```python
from build123d import *

# Parameters (mm, degrees)
SKETCH1_R           = 30
BOSS_EXTRUDE1_DEPTH = 3
SKETCH2_R           = 10
BOSS_EXTRUDE2_DEPTH = 2
SKETCH3_W           = 10
SKETCH3_H           = 15
BOSS_EXTRUDE3_DEPTH = 10
CUT_EXTRUDE1_START  = -1.5
SKETCH4_W           = 10
SKETCH4_H           = 10
CUT_EXTRUDE1_DEPTH  = 12
SKETCH5_R           = 2.5
CUT_EXTRUDE2_DEPTH  = 50.751884386


with BuildPart() as part:
    # Sketch1 → Boss-Extrude1 (new body)
    with BuildSketch(Plane(origin=(0, 0, 0), x_dir=(1, 0, 0), z_dir=(0, 1, 0))):
        with Locations(Location((0, 0, 0), (0, 0, 270))):
            Circle(SKETCH1_R)
    extrude(amount=BOSS_EXTRUDE1_DEPTH)

    # Sketch2 → Boss-Extrude2 (add)
    with BuildSketch(Plane(origin=(0, 3, 0), x_dir=(1, 0, 0), z_dir=(0, 1, 0))):
        with Locations(Location((0, 0, 0), (0, 0, 270))):
            Circle(SKETCH2_R)
    extrude(amount=BOSS_EXTRUDE2_DEPTH)

    # Sketch3 → Boss-Extrude3 (add)
    with BuildSketch(Plane(origin=(0, 3, 0), x_dir=(1, 0, 0), z_dir=(0, 1, 0))):
        with Locations((-20, 0)):
            Rectangle(SKETCH3_W, SKETCH3_H)
        with Locations((20, 0)):
            Rectangle(SKETCH3_W, SKETCH3_H)
    extrude(amount=BOSS_EXTRUDE3_DEPTH)

    # Sketch4 → Cut-Extrude1 (cut)
    with BuildSketch(Plane.XY.offset(7.5).offset(CUT_EXTRUDE1_START)):
        with Locations((-20, 8)):
            Rectangle(SKETCH4_W, SKETCH4_H)
        with Locations((20, 8)):
            Rectangle(SKETCH4_W, SKETCH4_H)
    extrude(amount=-CUT_EXTRUDE1_DEPTH, mode=Mode.SUBTRACT)

    # Sketch5 → Cut-Extrude2 (cut, through all)
    with BuildSketch(Plane.XY.offset(7.5)):
        with Locations((20, 8)):
            Circle(SKETCH5_R)
        with Locations((-20, 8)):
            Circle(SKETCH5_R)
    extrude(amount=-CUT_EXTRUDE2_DEPTH, mode=Mode.SUBTRACT)


solid = part.part
```
Geometry check sheet. Reference: the model listing, model coordinates, mm. A direction names the side the tool comes from. Coordinates: 2 decimals unless noted, no trailing zeros. Write each loop counter-clockwise with the first axis right and the second up, starting at its lowest first coordinate (ties: lowest second). Pieces come first, ordered by that corner, then holes. Notation, with made-up numbers: M 2.25,-30 L 37.25,-30 A10 ccw 37.25,-24 Z; hole C 13,13.5 d2. An arc over 180 degrees is marked long. One line per item, written item: value. Start each with the question number.
(1) Sectioned sample at B-B, the plane y = 4.25. Enter the section's corners in (x, z).
(2) Depth check by flat-ended pin: pin 1 (0.8 mm diameter, centred on y = 10, z = -7, fed in from -X); pin 2 (1.6 mm diameter, centred on y = 9.5, z = -7, fed in from +X); pin 3 (5 mm diameter, centred on y = 6.5, z = -3, fed in from -X). Enter the tip coordinate at first touch or a pass-through.
(3) Release check for a two-part mould opening along X. For faces 1 (the face through (-22, 6, -7.5)), 2 (the face through (-22, 6.5, 6.8)), 3 (the face through (-25, 8, 7)) record: released by +X, released by -X, zero draft, split by the parting line, or undercut.
(4) Tool access check on faces 4 (the face through (25, 8, -7)), 5 (the face through (18, 10, 6)), 6 (the face through (-15, 8, 7)), 7 (the face through (-22, 10, -6)). Record the directions out of +Z, -Z, +X, -X, +Y, -Y that give a thin tool (end or side, any length) a straight path to the whole face; none if there is none.
(5) Scan lines: line 1 along Y through (x, z) = (20, 7); line 2 along Z through (x, y) = (22, 6); line 3 along X through (y, z) = (12.25, -6.5). Record each from-to range of solid material in increasing order. Write a range as [from, to].
(6) Sectioned sample at D-D, the plane z = 0. Enter the section's corners in (x, y).
(7) Sectioned sample at C-C, the plane x = -20. Enter the section's corners in (y, z), and give its area (3 significant figures).
(8) Sectioned sample at A-A, the plane y = 11.75. Enter the section's corners in (x, z), and give its area (3 significant figures).
Filled sheet:
1. outline: M -25,-7.5 L -15,-7.5 L -15,-6 L -25,-6 Z; M -25,6 L -15,6 L -15,7.5 L -25,7.5 Z; C 0,0 d20; M 15,-7.5 L 25,-7.5 L 25,-6 L 15,-6 Z; M 15,6 L 25,6 L 25,7.5 L 15,7.5 Z
2. pin 1: x = -25
2. pin 2: x = 25
2. pin 3: x = -9.95
3. face 1: zero draft
3. face 2: undercut
3. face 3: released by -X
4. face 4: +Z, -Z, +X, +Y
4. face 5: +X, +Y
4. face 6: +Z, -Z, +Y
4. face 7: -X, +Y
5. line 1: [0, 5.5], [10.5, 13]
5. line 2: [-7.5, -6], [6, 7.5]
5. line 3: [-25, -15], [15, 25]
6. outline: M -30,0 L 30,0 L 30,3 L 10,3 L 10,5 L -10,5 L -10,3 L -30,3 Z
7. outline: M 0,-22.36 L 3,-22.36 L 3,-7.5 L 5.5,-7.5 L 5.5,-6 L 3,-6 L 3,6 L 5.5,6 L 5.5,7.5 L 3,7.5 L 3,22.36 L 0,22.36 Z; M 10.5,-7.5 L 13,-7.5 L 13,-6 L 10.5,-6 Z; M 10.5,6 L 13,6 L 13,7.5 L 10.5,7.5 Z
7. area: 149 mm²
8. outline: M -25,-7.5 L -15,-7.5 L -15,-6 L -25,-6 Z; M -25,6 L -15,6 L -15,7.5 L -25,7.5 Z; M 15,-7.5 L 25,-7.5 L 25,-6 L 15,-6 Z; M 15,6 L 25,6 L 25,7.5 L 15,7.5 Z
8. area: 60.0 mm²
